from build123d import *

# Parameters (mm, degrees)
F1_W          = 95.6
F1_H          = 48
F1_R          = 3
F1_R_2        = 1.75
F2_DEPTH      = 1.5
F1_W_2        = 97.6
F1_H_2        = 50
F3_DEPTH      = 25
F1_W_3        = 99.6
F1_H_3        = 52
F4_DEPTH      = 57
F5_R          = 2
F6_DEPTH      = 49.801
F6_DEPTH_BACK = 49.801
F7_SIZE       = 0.99999
F8_R          = 0.5


# Not quite as in the source:
# - a fillet or chamfer is up to 0.001 mm smaller than in the source, because OpenCascade refuses the exact size


with BuildPart() as f2:
    # F1 (on Top) → F2 (new body)
    with BuildSketch(Plane.XY):
        Rectangle(F1_W, F1_H)
        with Locations((-34.0166666667, 0)):
            Circle(F1_R, mode=Mode.SUBTRACT)
        with Locations((-20.2333333333, 0)):
            Circle(F1_R, mode=Mode.SUBTRACT)
        with Locations((-6.45, 0)):
            Circle(F1_R_2, mode=Mode.SUBTRACT)
        Polygon((-2.2, -13.3), (-2.2, 13.3), (35, 13.3), (40.3, 8), (40.3, -8), (35, -13.3), align=None, mode=Mode.SUBTRACT)
        with Locations((44.55, 0)):
            Circle(F1_R_2, mode=Mode.SUBTRACT)
    extrude(amount=F2_DEPTH)

    # F1 (on Top) → F3 (join)
    with BuildSketch(Plane.XY):
        Rectangle(F1_W_2, F1_H_2)
        Rectangle(F1_W, F1_H, mode=Mode.SUBTRACT)
    extrude(amount=F3_DEPTH)

    # F1 (on Top) → F4 (join)
    with BuildSketch(Plane.XY):
        Rectangle(F1_W_3, F1_H_3)
        Rectangle(F1_W_2, F1_H_2, mode=Mode.SUBTRACT)
    extrude(amount=F4_DEPTH)

    # F5 (on Right) → F6 (cut, two sides)
    with BuildSketch(Plane.YZ) as f6_sk:
        with Locations((13.5, 50)):
            Circle(F5_R)
    extrude(amount=-F6_DEPTH, mode=Mode.SUBTRACT)
    extrude(f6_sk.sketch, amount=F6_DEPTH_BACK, mode=Mode.SUBTRACT)

    # F7 (size 1 in the source; OpenCascade refuses exactly that, so slightly less here)
    f7_edges = [f2.edges().sort_by_distance(p)[0] for p in [
        (49.8, 11.5, 50),
        (-49.8, 11.5, 50),
    ]]
    chamfer(f7_edges, length=F7_SIZE)

    # F8
    f8_edges = [f2.edges().sort_by_distance(p)[0] for p in [
        (-17.233333, 0, 0.75),
        (-23.233333, 0, 0),
        (-23.233333, 0, 1.5),
        (-31.016667, 0, 0.75),
        (-37.016667, 0, 0),
        (-37.016667, 0, 1.5),
        (-47.8, 0, 1.5),
        (0, 24, 1.5),
        (47.8, 0, 1.5),
        (47.8, 24, 13.25),
        (-47.8, 24, 13.25),
        (-47.8, -24, 13.25),
        (0, -24, 1.5),
        (47.8, -24, 13.25),
    ]]
    fillet(f8_edges, radius=F8_R)


solid = f2.part
Design review of the part built by this model. Coordinates are the model's own, in mm. A direction names the side the tool comes from. Coordinates: 2 decimals unless noted, no trailing zeros. Order: outer loops, then holes, each group sorted by start corner. A loop starts at its lowest first (then second) coordinate and runs counter-clockwise, first axis right, second up.
Item 1: Take a section at C-C, the plane z = 37. Write out the cut boundary in (x, y).
Item 2: For line 1 (X direction, y = -0.5, z = 21); line 2 (Y direction, x = 45, z = 5); line 3 (Y direction, x = -48, z = 50), list the stretches that pass through material, from the lowest coordinate up.
Item 3: Take a section at D-D, the plane y = 0. Count the separate pieces of the cut face and the enclosed holes in it, then the cut area to 3 significant figures.
Item 4: Take a section at B-B, the plane x = 44.55. Write out the cut boundary in (y, z).
Item 5: For pin 1 Ø3 at (x, y) = (-6.45, 0) entering from +Z; pin 2 Ø5 at (y, z) = (13.5, 50) entering from +X; pin 3 Ø8 at (x, y) = (-20.23, 0) entering from -Z, all flat-tipped, find the tip position at first contact; note any pin that passes through.
Item 6: For faces 1 (the flat face through (37.7, -10.6, 0.7)), 2 (the flat face through (-0.2, 25.2, 57)), 3 (the flat face through (-0.2, 24.2, 25)), list the 3-axis set-ups (+Z, -Z, +X, -X, +Y, -Y) from which the entire face can be reached by the end or side of a thin tool; tool diameter is ignored.
The answers:
1. outline: (-49.8, -26) - (49.8, -26) - (49.8, 26) - (-49.8, 26) - close; hole (-48.8, -25) - (48.8, -25) - (48.8, 25) - (-48.8, 25) - close
2. line 1: x = -49.8 to -47.8, 47.8 to 49.8
2. line 2: y = -26 to -24, 24 to 26
2. line 3: y = -26 to -25, 25 to 26
3. separate pieces: 6
3. enclosed holes: 0
3. area: 215 mm2
4. outline: (-26, 0) - (-1.75, 0) - (-1.75, 1.5) - (-23.5, 1.5) arc R0.5 cw to (-24, 2) - (-24, 25) - (-25, 25) - (-25, 57) - (-26, 57) - close; (1.75, 0) - (26, 0) - (26, 57) - (25, 57) - (25, 25) - (24, 25) - (24, 2) arc R0.5 cw to (23.5, 1.5) - (1.75, 1.5) - close
5. pin 1: passes through
5. pin 2: stops at x = 49.3
5. pin 3: stops at z = 0
6. face 1: +Z, -Z
6. face 2: +Z, +X, -X, +Y, -Y
6. face 3: +Z
